from build123d import *

# Parameters (mm, degrees)
SZKIC1_W                    = 36
SZKIC1_H                    = 18
DODANIE_WYCI_GNI_CIE1_DEPTH = 9
WYTNIJ_WYCI_GNI_CIE1_DEPTH  = 18
SZKIC3_R                    = 1.182612818
DODANIE_WYCI_GNI_CIE2_DEPTH = 18
WYTNIJ_WYCI_GNI_CIE2_DEPTH  = 40


with BuildPart() as part:
    # Szkic1 → Dodanie-wyciągnięcie1 (new, symmetric)
    with BuildSketch(Plane.XY):
        Rectangle(SZKIC1_W, SZKIC1_H)
    extrude(amount=DODANIE_WYCI_GNI_CIE1_DEPTH, both=True)

    # Szkic2 → Wytnij-wyciągnięcie1 (cut)
    with BuildSketch(Plane.XZ.offset(9)):
        Polygon((-2, 9), (4, 3), (18, 3), (18, 9), align=None)
    extrude(amount=-WYTNIJ_WYCI_GNI_CIE1_DEPTH, mode=Mode.SUBTRACT)

    # Szkic3 → Dodanie-wyciągnięcie2 (add)
    with BuildSketch(Plane(origin=(18, 0, 0), x_dir=(0, 0, -1), z_dir=(1, 0, 0))):
        with Locations(Location((0, 0, 0), (0, 0, 180))):
            Circle(SZKIC3_R)
    extrude(amount=DODANIE_WYCI_GNI_CIE2_DEPTH)

    # Szkic4 → Wytnij-wyciągnięcie2 (cut, through all)
    with BuildSketch(Plane.XY.offset(3)):
        with BuildLine():
            Line((7, 6.85), (14, 6.85))
            ThreePointArc((14, 6.85), (15.6, 5.25), (14, 3.65))
            Line((14, 3.65), (7, 3.65))
            ThreePointArc((7, 3.65), (5.4, 5.25), (7, 6.85))
        make_face()
        with BuildLine():
            Line((7, -6.85), (14, -6.85))
            ThreePointArc((14, -6.85), (15.6, -5.25), (14, -3.65))
            Line((14, -3.65), (7, -3.65))
            ThreePointArc((7, -3.65), (5.4, -5.25), (7, -6.85))
        make_face()
    extrude(amount=-WYTNIJ_WYCI_GNI_CIE2_DEPTH, mode=Mode.SUBTRACT)


solid = part.part
Work out the finished part from the listing and answer in its coordinate system (mm). A direction names the side the tool comes from. Coordinates: 2 decimals unless noted, no trailing zeros. Loops run counter-clockwise (first coordinate to the right, second up) from the corner with the lowest first, then second, coordinate; pieces in that order, holes last. Notation, with made-up numbers: M 32,33.25 L 50,33.25 A25 ccw 50,45.25 Z; hole C 13.25,66.25 d3. An arc over 180 degrees is marked long. Answer in a Markdown table with one row per item. Add a question column.
1. Find section D-D, the plane x = 15. Write down the section's boundary in (y, z).
2. Flat-ended cylindrical pins translate along their axes: P1, Ø5, axis at x = 22, y = 1.5, coming from the -Z side; P2, Ø1, axis at y = -1, z = -6, coming from the +X side; P3, Ø8, axis at x = 13, y = 0.5, coming from the +Z side. Find the tip coordinate at first contact, or state that the pin passes through.
3. Find section B-B, the plane y = -5.25. Write down the section's boundary in (x, z).
4. A tool of negligible diameter and unlimited length cuts with its end or side. For faces 1 (the cylindrical face through (26.87, 0.72, -0.94)), 2 (the flat face through (11, 0, 3)), 3 (the flat face through (0, -9, -2)), 4 (the cylindrical face through (15.6, 5.3, -2.9)), 5 (the flat face through (0, 9, -2)), from which of +Z, -Z, +X, -X, +Y, -Y can it reach the whole face along a straight path? Write none if from no direction.
5. Find section A-A, the plane z = 0. Write down the section's boundary in (x, y).
6. Consider L1, parallel to Z at x = 12, y = -7.75; L2, parallel to X at y = 0, z = 2.5; L3, parallel to X at y = 0.75, z = 4.25. Determine where each line is inside the solid, lowest interval first.
7. The mould has two halves that part along X. Classify faces 6 (the cylindrical face through (5.4, 5.2, -2.9)), 7 (the flat face through (1, 0, 6)), 8 (the flat face through (11, -3.65, -3)), 9 (the flat face through (0, 0, -9)): pulls with the +X half, pulls with the -X half, needs draft (parallel to the pull), parting line crosses it, or undercut.
8. Find section C-C, the plane y = 0. Write down the section's boundary in (x, z), then the cut area to 3 significant figures.
Reported:
| question | item | result |
|---|---|---|
| 1 | outline | M -9,-9 L -6.5,-9 L -6.5,3 L -9,3 Z; M -4,-9 L 4,-9 L 4,3 L -4,3 Z; M 6.5,-9 L 9,-9 L 9,3 L 6.5,3 Z |
| 2 | P1 | stops at z = -1.18 |
| 2 | P2 | stops at x = 18 |
| 2 | P3 | stops at z = 3 |
| 3 | outline | M -18,-9 L 5.4,-9 L 5.4,3 L 4,3 L -2,9 L -18,9 Z; M 15.6,-9 L 18,-9 L 18,3 L 15.6,3 Z |
| 4 | face 1 | +X |
| 4 | face 2 | +Z, +X, +Y, -Y |
| 4 | face 3 | +Z, -Z, +X, -X, -Y |
| 4 | face 4 | +Z, -Z |
| 4 | face 5 | +Z, -Z, +X, -X, +Y |
| 5 | outline | M -18,-9 L 18,-9 L 18,-1.18 L 36,-1.18 L 36,1.18 L 18,1.18 L 18,9 L -18,9 Z; hole M 7,-6.85 L 14,-6.85 A1.6 ccw 14,-3.65 L 7,-3.65 A1.6 ccw Z; hole M 7,3.65 L 14,3.65 A1.6 ccw 14,6.85 L 7,6.85 A1.6 ccw Z |
| 6 | L1 | z = -9 to 3 |
| 6 | L2 | x = -18 to 18 |
| 6 | L3 | x = -18 to 2.75 |
| 7 | face 6 | undercut |
| 7 | face 7 | pulls with the +X half |
| 7 | face 8 | undercut |
| 7 | face 9 | needs draft |
| 8 | outline | M -18,-9 L 18,-9 L 18,-1.18 L 36,-1.18 L 36,1.18 L 18,1.18 L 18,3 L 4,3 L -2,9 L -18,9 Z |
| 8 | area | 589 mm^2 |
